from build123d import *

# Parameters (mm, degrees)
EXTRUDE_1_DEPTH     = 3
SKETCH_5_R          = 2.1
CUT_EXTRUDE_4_DEPTH = 240
CHAMFER_2_SIZE      = 2.5


with BuildPart() as part:
    # 草图1 → 凸台-拉伸1 (new, symmetric)
    with BuildSketch(Plane(origin=(0, 0, 0), x_dir=(1, 0, 0), z_dir=(0, 1, 0))):
        with BuildLine():
            Line((-150, -140), (150, -140))
            ThreePointArc((150, -140), (157.071067812, -137.071067812), (160, -130))
            Line((160, -130), (160, 130))
            ThreePointArc((160, 130), (157.071067812, 137.071067812), (150, 140))
            Line((150, 140), (-150, 140))
            ThreePointArc((-150, 140), (-157.071067812, 137.071067812), (-160, 130))
            Line((-160, 130), (-160, -130))
            ThreePointArc((-160, -130), (-157.071067812, -137.071067812), (-150, -140))
        make_face()
    extrude(amount=EXTRUDE_1_DEPTH, both=True)

    # 草图5 → 切除-拉伸4 (cut)
    with BuildSketch(Plane(origin=(0, 3, 0), x_dir=(1, 0, 0), z_dir=(0, 1, 0))):
        with Locations(Location((0, 60, 0), (0, 0, 270))):
            Circle(SKETCH_5_R)
        with Locations(Location((40, 60, 0), (0, 0, 270))):
            Circle(SKETCH_5_R)
        with Locations(Location((80, 60, 0), (0, 0, 270))):
            Circle(SKETCH_5_R)
        with Locations(Location((120, 60, 0), (0, 0, 270))):
            Circle(SKETCH_5_R)
        with Locations(Location((-120, 60, 0), (0, 0, 270))):
            Circle(SKETCH_5_R)
        with Locations(Location((-80, 60, 0), (0, 0, 270))):
            Circle(SKETCH_5_R)
        with Locations(Location((-40, 60, 0), (0, 0, 270))):
            Circle(SKETCH_5_R)
        with Locations(Location((-40, -60, 0), (0, 0, 270))):
            Circle(SKETCH_5_R)
        with Locations(Location((-80, -60, 0), (0, 0, 270))):
            Circle(SKETCH_5_R)
        with Locations(Location((-120, -60, 0), (0, 0, 270))):
            Circle(SKETCH_5_R)
        with Locations(Location((120, -60, 0), (0, 0, 270))):
            Circle(SKETCH_5_R)
        with Locations(Location((80, -60, 0), (0, 0, 270))):
            Circle(SKETCH_5_R)
        with Locations(Location((40, -60, 0), (0, 0, 270))):
            Circle(SKETCH_5_R)
        with Locations(Location((0, -60, 0), (0, 0, 270))):
            Circle(SKETCH_5_R)
        with Locations(Location((-150, 0, 0), (0, 0, 270))):
            Circle(SKETCH_5_R)
        with Locations(Location((-150, -40, 0), (0, 0, 270))):
            Circle(SKETCH_5_R)
        with Locations(Location((-150, -80, 0), (0, 0, 270))):
            Circle(SKETCH_5_R)
        with Locations(Location((-150, 80, 0), (0, 0, 270))):
            Circle(SKETCH_5_R)
        with Locations(Location((-150, 40, 0), (0, 0, 270))):
            Circle(SKETCH_5_R)
        with Locations(Location((150, 40, 0), (0, 0, 270))):
            Circle(SKETCH_5_R)
        with Locations(Location((150, 80, 0), (0, 0, 270))):
            Circle(SKETCH_5_R)
        with Locations(Location((150, -80, 0), (0, 0, 270))):
            Circle(SKETCH_5_R)
        with Locations(Location((150, -40, 0), (0, 0, 270))):
            Circle(SKETCH_5_R)
        with Locations(Location((150, 0, 0), (0, 0, 270))):
            Circle(SKETCH_5_R)
    extrude(amount=-CUT_EXTRUDE_4_DEPTH, mode=Mode.SUBTRACT)

    # 倒角2
    chamfer_2_edges = [part.edges().sort_by_distance(p)[0] for p in [
        (-80, 3, -62.1),
        (-40, 3, -62.1),
        (-40, 3, 57.9),
        (-150, 3, -82.1),
        (-150, 3, -42.1),
        (150, 3, -42.1),
        (150, 3, -82.1),
        (150, 3, 77.9),
        (150, 3, 37.9),
        (150, 3, -2.1),
        (0, 3, -62.1),
        (-80, 3, 57.9),
        (-120, 3, 57.9),
        (120, 3, 57.9),
        (80, 3, 57.9),
        (40, 3, 57.9),
        (0, 3, 57.9),
        (-150, 3, 37.9),
        (-150, 3, 77.9),
        (-150, 3, -2.1),
        (120, 3, -62.1),
        (80, 3, -62.1),
        (40, 3, -62.1),
        (-120, 3, -62.1),
    ]]
    chamfer(chamfer_2_edges, length=CHAMFER_2_SIZE)


solid = part.part
Could you check a few things on this model? Use its own coordinates, in mm. Round coordinates to 2 decimals unless told otherwise and drop trailing zeros. Use a Markdown table: item, result.
Q1. For pin 1 (5 mm diameter, centred on x = -40, z = -60, fed in from +Y); pin 2 (6.5 mm diameter, centred on x = -40, z = 60, fed in from +Y), each with a flat end and sliding along its axis, tell me the tip position at first contact or that it passes through.
Output values:
| item | result |
|---|---|
| pin 1 | y = 0.9 |
| pin 2 | y = 1.65 |
Q2. Please list where these lines run through material, in increasing order: L1, parallel to Z at x = -150, y = -1.8; L2, parallel to X at y = -0.75, z = -40; L3, parallel to Z at x = -41.5, y = 1.75.
Output values:
| item | result |
|---|---|
| L1 | -140 to -82.1, -77.9 to -42.1, -37.9 to -2.1, 2.1 to 37.9, 42.1 to 77.9, 82.1 to 140 |
| L2 | -160 to -152.1, -147.9 to 147.9, 152.1 to 160 |
| L3 | -140 to -63, -57 to 57, 63 to 140 |
Q3. Thinking about a two-plate mould opening in X: for faces 1 (the conical face through (39.15, 0.62, -57.95)), 2 (the cylindrical face through (-157.15, 0.04, 136.99)), 3 (the flat face through (-2, -3, -2)), which applies, released by +X, released by -X, zero draft, split by the parting line, or undercut?
Output values:
| item | result |
|---|---|
| face 1 | undercut |
| face 2 | released by -X |
| face 3 | zero draft |
